```python
from build123d import *

# Parameters (mm, degrees)
SKETCH1_R           = 10.8
SKETCH1_R_2         = 2.7
BOSS_EXTRUDE1_DEPTH = 11.5
BOSS_EXTRUDE3_START = 1
BOSS_EXTRUDE3_DEPTH = 9.5


with BuildPart() as part:
    # Sketch1 → Boss-Extrude1 (new body)
    with BuildSketch(Plane(origin=(0, 0, 0), x_dir=(1, 0, 0), z_dir=(0, 1, 0))):
        Circle(SKETCH1_R)
        with Locations(Location((0, 0, 0), (0, 0, 270))):
            Circle(SKETCH1_R_2, mode=Mode.SUBTRACT)
        with BuildLine():
            ThreePointArc((-8.026244712, 7.226298902), (-6.348080725, 8.737383539), (-4.392372642, 9.866461502))
            Line((-4.392372642, 9.866461502), (-6.806272613, 11.494657591))
            Line((-6.806272613, 11.494657591), (-8.828815098, 10.02519446))
            Line((-8.828815098, 10.02519446), (-8.026244712, 7.226298902))
        make_face()
        with BuildLine():
            ThreePointArc((-10.740880296, 1.128490345), (-10.271410376, 3.337383539), (-9.352864677, 5.400363168))
            Line((-9.352864677, 5.400363168), (-12.262780424, 5.298746671))
            Line((-12.262780424, 5.298746671), (-13.03532291, 2.92110538))
            Line((-13.03532291, 2.92110538), (-10.740880296, 1.128490345))
        make_face()
        with BuildLine():
            ThreePointArc((-9.352864677, -5.400363168), (-10.271410376, -3.337383539), (-10.740880296, -1.128490345))
            Line((-10.740880296, -1.128490345), (-13.03532291, -2.92110538))
            Line((-13.03532291, -2.92110538), (-12.262780424, -5.298746671))
            Line((-12.262780424, -5.298746671), (-9.352864677, -5.400363168))
        make_face()
        with BuildLine():
            ThreePointArc((-4.392372642, -9.866461502), (-6.348080725, -8.737383539), (-8.026244712, -7.226298902))
            Line((-8.026244712, -7.226298902), (-8.828815098, -10.02519446))
            Line((-8.828815098, -10.02519446), (-6.806272613, -11.494657591))
            Line((-6.806272613, -11.494657591), (-4.392372642, -9.866461502))
        make_face()
        with BuildLine():
            ThreePointArc((0, -10.8), (-1.129115932, -10.740814551), (-2.24585645, -10.563906891))
            Line((-2.24585645, -10.563906891), (-1.25, -13.3))
            Line((-1.25, -13.3), (1.25, -13.3))
            Line((1.25, -13.3), (2.159925586, -10.8))
            Line((2.159925586, -10.8), (0, -10.8))
        make_face()
        with BuildLine():
            Line((8.828815098, -10.02519446), (8.026244712, -7.226298902))
            ThreePointArc((8.026244712, -7.226298902), (6.348080725, -8.737383539), (4.392372642, -9.866461502))
            Line((4.392372642, -9.866461502), (5.776400382, -10.8))
            Line((5.776400382, -10.8), (7.762386761, -10.8))
            Line((7.762386761, -10.8), (8.828815098, -10.02519446))
        make_face()
        Polygon((6.806272613, -11.494657591), (7.762386761, -10.8), (5.776400382, -10.8), align=None)
        with BuildLine():
            Line((13.03532291, -2.92110538), (10.740880296, -1.128490345))
            ThreePointArc((10.740880296, -1.128490345), (10.271410376, -3.337383539), (9.352864677, -5.400363168))
            Line((9.352864677, -5.400363168), (12.262780424, -5.298746671))
            Line((12.262780424, -5.298746671), (13.03532291, -2.92110538))
        make_face()
        with BuildLine():
            Line((12.262780424, 5.298746671), (9.352864677, 5.400363168))
            ThreePointArc((9.352864677, 5.400363168), (9.996560411, 4.087637453), (10.457055035, 2.7))
            Line((10.457055035, 2.7), (12.752320929, 2.7))
            Line((12.752320929, 2.7), (13.03532291, 2.92110538))
            Line((13.03532291, 2.92110538), (12.262780424, 5.298746671))
        make_face()
        with BuildLine():
            Line((12.752320929, 2.7), (10.457055035, 2.7))
            ThreePointArc((10.457055035, 2.7), (10.628053736, 1.919498314), (10.740880296, 1.128490345))
            Line((10.740880296, 1.128490345), (12.752320929, 2.7))
        make_face()
        with BuildLine():
            Line((1.25, 13.3), (-1.25, 13.3))
            Line((-1.25, 13.3), (-2.24585645, 10.563906891))
            ThreePointArc((-2.24585645, 10.563906891), (0, 10.8), (2.24585645, 10.563906891))
            Line((2.24585645, 10.563906891), (1.25, 13.3))
        make_face()
        with BuildLine():
            Line((6.806272613, 11.494657591), (4.392372642, 9.866461502))
            ThreePointArc((4.392372642, 9.866461502), (6.348080725, 8.737383539), (8.026244712, 7.226298902))
            Line((8.026244712, 7.226298902), (8.828815098, 10.02519446))
            Line((8.828815098, 10.02519446), (6.806272613, 11.494657591))
        make_face()
        with BuildLine():
            ThreePointArc((2.24585645, -10.563906891), (1.129115932, -10.740814551), (0, -10.8))
            Line((0, -10.8), (2.159925586, -10.8))
            Line((2.159925586, -10.8), (2.24585645, -10.563906891))
        make_face()
    extrude(amount=BOSS_EXTRUDE1_DEPTH)

    # Sketch1_4 → Boss-Extrude3 (add)
    with BuildSketch(Plane(origin=(0, 0, 0), x_dir=(1, 0, 0), z_dir=(0, 1, 0)).offset(BOSS_EXTRUDE3_START)):
        with BuildLine():
            Line((18.412545051, 2.7), (12.752320929, 2.7))
            Line((12.752320929, 2.7), (10.740880296, 1.128490345))
            ThreePointArc((10.740880296, 1.128490345), (10.785209947, 0.565018937), (10.8, 0))
            ThreePointArc((10.8, 0), (10.785209947, -0.565018937), (10.740880296, -1.128490345))
            Line((10.740880296, -1.128490345), (13.03532291, -2.92110538))
            Line((13.03532291, -2.92110538), (12.262780424, -5.298746671))
            Line((12.262780424, -5.298746671), (9.352864677, -5.400363168))
            ThreePointArc((9.352864677, -5.400363168), (8.737383539, -6.348080725), (8.026244712, -7.226298902))
            Line((8.026244712, -7.226298902), (8.828815098, -10.02519446))
            Line((8.828815098, -10.02519446), (7.762386761, -10.8))
            Line((7.762386761, -10.8), (29.369189077, -10.8))
            ThreePointArc((29.369189077, -10.8), (30.646867306, -10.338680715), (31.335127928, -9.167538342))
            ThreePointArc((31.335127928, -9.167538342), (51.109657071, 7.156746799), (70.69491969, -9.394137658))
            ThreePointArc((70.69491969, -9.394137658), (71.19716993, -9.807823175), (71.682924587, -9.374887357))
            ThreePointArc((71.682924587, -9.374887357), (51.897130707, 20.096844573), (20.274570163, 3.970025697))
            ThreePointArc((20.274570163, 3.970025697), (19.539499219, 3.047736612), (18.412545051, 2.7))
        make_face()
    extrude(amount=BOSS_EXTRUDE3_DEPTH)


solid = part.part
```
Verification items for the finished model (mm, model axes). A direction names the side the tool comes from. Coordinates: 2 decimals unless noted, no trailing zeros. Loops run counter-clockwise (first coordinate to the right, second up) from the corner with the lowest first, then second, coordinate; pieces in that order, holes last. Notation, with made-up numbers: (45, 8.25) -> (53, 8.25) arc R32 ccw to (53, 36.25) -> close; hole circle Ø2 at (66, -36.5). An arc over 180 degrees is marked (long way). Put each result on its own line as item: value.
1. Mould release check, pull along X, two halves, no side actions. Record for faces 1 (the face through (1.755, 5.67, -11.913)), 2 (the face through (39, 10.5, -5)), 3 (the face through (-7.803, 5.67, -10.77)): pulls with the +X half, pulls with the -X half, needs draft (parallel to the pull), parting line crosses it, or undercut.
Result set:
face 1: undercut
face 2: needs draft
face 3: pulls with the -X half
2. Section check C-C, the plane x = 14. Record the boundary of the cut face in (y, z), then the cut area to 3 significant figures.
Result set:
outline: (1, -2.7) -> (10.5, -2.7) -> (10.5, 10.8) -> (1, 10.8) -> close
area: 128 mm^2
3. Section check D-D, the plane x = 59.5. Record the boundary of the cut face in (y, z), then the cut area to 3 significant figures.
Result set:
outline: (1, -16.8) -> (10.5, -16.8) -> (10.5, -5.26) -> (1, -5.26) -> close
area: 110 mm^2
4. Gauge pin test, flat ends, axial feed: P1, Ø3, axis at x = 24.5, y = 1.5, coming from the -Z side; P2, Ø3, axis at y = 8, z = -5.5, coming from the +X side; P3, Ø4, axis at y = 3, z = 4, coming from the +X side. Record the tip position at first contact, or that the pin passes through.
Result set:
P1: stops at z = -12.85
P2: stops at x = 70.07
P3: stops at x = 71.92
5. Section check A-A, the plane x = 0. Record the boundary of the cut face in (y, z), then the cut area to 3 significant figures.
Result set:
outline: (0, -13.3) -> (11.5, -13.3) -> (11.5, -2.7) -> (0, -2.7) -> close; (0, 2.7) -> (11.5, 2.7) -> (11.5, 13.3) -> (0, 13.3) -> close
area: 244 mm^2
6. Tool access check on faces 4 (the face through (-11.87, 5.67, 2.01)), 5 (the face through (11.904, 10.993, 2.037)), 6 (the face through (3.322, 5.67, 10.276)), 7 (the face through (-3.322, 5.67, -10.276)). Record the directions out of +Z, -Z, +X, -X, +Y, -Y that give a thin tool (end or side, any length) a straight path to the whole face; none if there is none.
Result set:
face 4: -X, +Y, -Y
face 5: +X, +Y
face 6: +Z, +Y, -Y
face 7: -Z, +Y, -Y
7. Thickness scan on line 1 (X direction, y = 1.25, z = 1); line 2 (X direction, y = 2.5, z = 0); line 3 (Y direction, x = 47, z = -8.5). Record the ranges inside material, lowest first.
Result set:
line 1: x = -10.75 to -2.51, 2.51 to 34.88, 67.11 to 71.49
line 2: x = -10.8 to -2.7, 2.7 to 35.66, 66.33 to 71.29
line 3: y = 1 to 10.5
8. Section check B-B, the plane z = 0. Record the boundary of the cut face in (x, y), then the cut area to 3 significant figures.
Result set:
outline: (-10.8, 0) -> (-2.7, 0) -> (-2.7, 11.5) -> (-10.8, 11.5) -> close; (2.7, 0) -> (10.8, 0) -> (10.8, 1) -> (35.66, 1) -> (35.66, 10.5) -> (10.8, 10.5) -> (10.8, 11.5) -> (2.7, 11.5) -> close; (66.33, 1) -> (71.29, 1) -> (71.29, 10.5) -> (66.33, 10.5) -> close
area: 470 mm^2
